For this review, use the dimensioned drawing (mm, ordinates from the lowest corner) and the shaded views. A direction names the side the tool comes from. Give positions to 0.01 mm unless a question says otherwise; leave off trailing zeros. Order: outer loops, then holes, each group sorted by start corner. A loop starts at its lowest first (then second) coordinate and runs counter-clockwise, first axis right, second up.
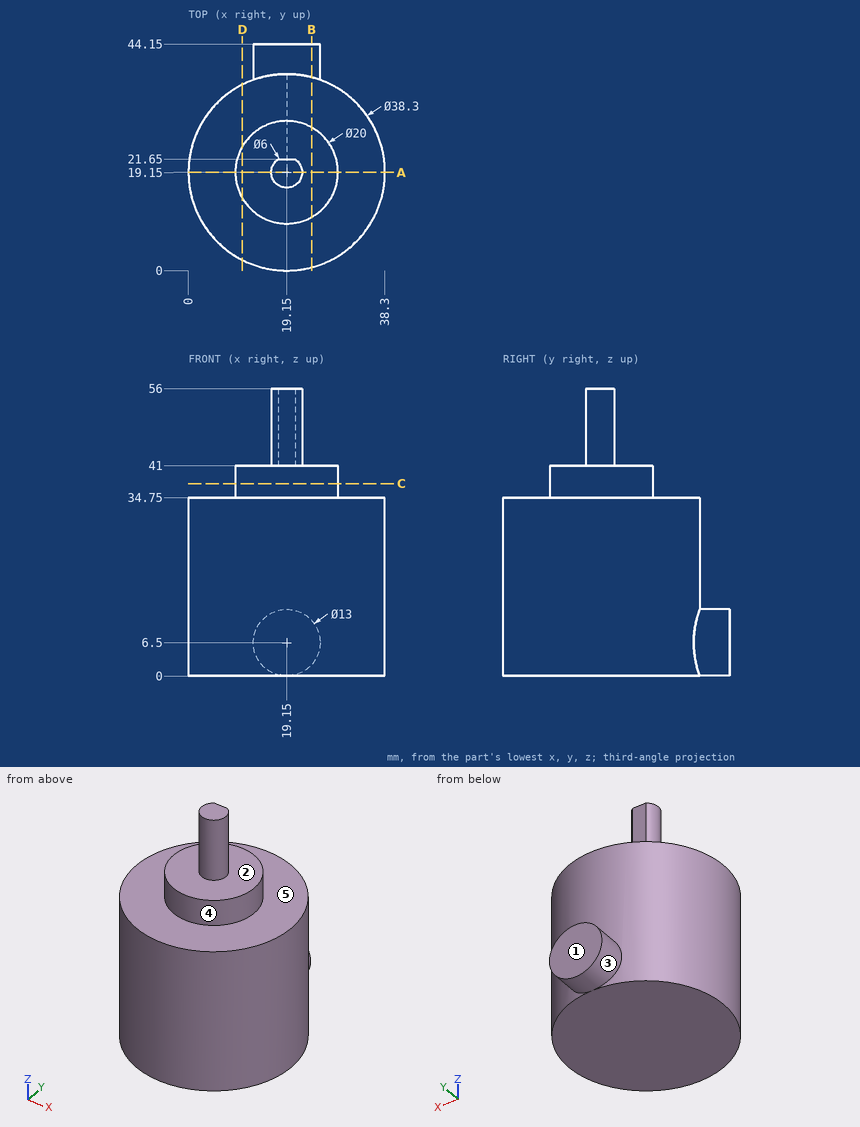
1. Take a section at D-D (x = 10.5). State the section outline as (y, z) points, then the cut area to 3 significant figures.
Recorded:
outline: (2.06, 0) - (36.24, 0) - (36.24, 34.75) - (24.17, 34.75) - (24.17, 41) - (14.13, 41) - (14.13, 34.75) - (2.06, 34.75) - close
area: 1,250 mm2
2. Take a section at C-C (z = 37.5). State the section outline as (x, y) points, then the cut area to 3 significant figures.
Recorded:
outline: circle Ø20 at (19.15, 19.15)
area: 314 mm2
3. Take a section at B-B (x = 24). State the section outline as (y, z) points.
Recorded:
outline: (0.62, 0) - (37.68, 0) - (37.68, 2.17) - (44.15, 2.17) - (44.15, 10.83) - (37.68, 10.83) - (37.68, 34.75) - (27.9, 34.75) - (27.9, 41) - (10.4, 41) - (10.4, 34.75) - (0.62, 34.75) - close
4. Draft analysis for pull direction X (two halves, no side actions). For the marked faces 4 and 5, state which applies: pulls with the +X half, pulls with the -X half, needs draft (parallel to the pull), parting line crosses it, or undercut.
Recorded:
face 4: parting line crosses it
face 5: needs draft
5. Take a section at A-A (y = 19.15). State the section outline as (x, z) points, then the cut area to 3 significant figures.
Recorded:
outline: (0, 0) - (38.3, 0) - (38.3, 34.75) - (29.15, 34.75) - (29.15, 41) - (22.15, 41) - (22.15, 56) - (16.15, 56) - (16.15, 41) - (9.15, 41) - (9.15, 34.75) - (0, 34.75) - close
area: 1,550 mm2
6. Machinability: for the marked faces 1, 2 and 3, which of the approach directions +Z, -Z, +X, -X, +Y, -Y give a long, thin tool a straight path to every point of the face, cutting with its end or side? Answer none if there is none.
Recorded:
face 1: +Z, -Z, +X, -X, +Y
face 2: +Z
face 3: +Y
7. For line 1 along Z through (x, y) = (32, 13); line 2 along Z through (x, y) = (25.5, 25.5); line 3 along X through (y, z) = (33, 23), list the stretches that pass through material, from the lowest coordinate up.
Recorded:
line 1: z = 0 to 34.75
line 2: z = 0 to 41
line 3: x = 5.93 to 32.37
8. For pin 1 (3 mm diameter, centred on x = 7, z = 36, fed in from -Y); pin 2 (1.7 mm diameter, centred on x = 18.5, z = 50, fed in from +Y); pin 3 (5 mm diameter, centred on x = 12.5, y = 25, fed in from +Z), all flat-tipped, find the tip position at first contact; note any pin that passes through.
Recorded:
pin 1: stops at y = 3.7
pin 2: stops at y = 21.65
pin 3: stops at z = 41
